Autodesk Inventor part; units mm, degrees
ref_plane "Work Plane1" through (-29.1, -14.5, 2.4) normal (0, 0, -1) x (0, 1, 0)
ref_plane "Work Plane2" through (-13.8999, -10.5497, 2.25) normal (0, 0, -1) x (0, 1, 0)
ref_plane "YZ Plane" through (0, 0, 0) normal (1, 0, 0) x (0, 1, 0)
ref_plane "Work Plane1" through (-29.1, -14.5, 2.4) normal (0, 0, -1) x (0, 1, 0)
ref_plane "Work Plane2" through (-13.8999, -10.5497, 2.25) normal (0, 0, -1) x (0, 1, 0)
sketch "Sketch1" plane through (0, 0, 0) normal (0, 0, 1) x (1, 0, 0)
  line L0 (-34.86, 0) -> (34.86, 0) construction
  line L1 (0, -34.86) -> (0, 34.86) construction
  line L2 (0, 0) -> (11.1575, 11.1575) construction
  line L3 (0, 0) -> (15.7791, 0) construction
  line L4 (0, 24.9) -> (16.8009, 24.9)
  line L5 (16.8009, 24.9) -> (16.8009, 21.2415)
  line L6 (16.8009, 21.2415) -> (19.0212, 19.0212)
  line L7 (24.9, 0) -> (24.9, 16.8009)
  line L8 (24.9, 16.8009) -> (21.2415, 16.8009)
  line L9 (21.2415, 16.8009) -> (19.0212, 19.0212)
  line L10 (0, -24.9) -> (16.8009, -24.9)
  line L11 (16.8009, -24.9) -> (16.8009, -21.2415)
  line L12 (16.8009, -21.2415) -> (19.0212, -19.0212)
  line L13 (24.9, 0) -> (24.9, -16.8009)
  line L14 (24.9, -16.8009) -> (21.2415, -16.8009)
  line L15 (21.2415, -16.8009) -> (19.0212, -19.0212)
  line L16 (0, 24.9) -> (-16.8009, 24.9)
  line L17 (-16.8009, 24.9) -> (-16.8009, 21.2415)
  line L18 (-16.8009, 21.2415) -> (-19.0212, 19.0212)
  line L19 (-24.9, 16.8009) -> (-21.2415, 16.8009)
  line L20 (-21.2415, 16.8009) -> (-19.0212, 19.0212)
  line L21 (0, -24.9) -> (-16.8009, -24.9)
  line L22 (-16.8009, -24.9) -> (-16.8009, -21.2415)
  line L23 (-16.8009, -21.2415) -> (-19.0212, -19.0212)
  line L24 (-21.2415, -16.8009) -> (-19.0212, -19.0212)
  line L25 (-24.9, -16.8009) -> (-21.2415, -16.8009)
  line L26 (-24.9, 0) -> (-24.9, -16.8009)
  line L27 (-24.9, 0) -> (-24.9, 16.8009)
  circle A0 centre (0, 0) radius 5
  dimension "d0" = 45
  dimension "d2" = 24.9
  dimension "d3" = 3.14
  dimension "d4" = 26.9
  dimension "d5" = 10
extrude "Extrusion1" add sketch "Sketch1" along normal up to surface (2.25 mm away)
sketch "Sketch5" plane through (0, 0, 0) normal (0, 0, -1) x (-1, 0, 0)
  circle A0 centre (-9.7, 10) radius 1.4
  circle A1 centre (-9.7, -10) radius 1.4
  circle A2 centre (13.8, 0) radius 1.4
  circle A3 centre (-10, 6.9) radius 0.75
  circle A4 centre (10, 6.9) radius 1.25
  point P0 (0, 0)
hole "Hole1" at (9.7, -10, 0) at (9.7, 10, 0) direction (0, 0, 1) diameter 3.3 depth 12 tip angle 118
sketch "Sketch6" plane through (-16.8009, 24.9, 2.25) normal (0, 0, 1) x (1, 0, 0)
  circle A0 centre (26.5009, -34.9) radius 1.65 construction
  circle A1 centre (26.5009, -14.9) radius 1.65 construction
  circle A2 centre (16.8009, -24.9) radius 5 construction
  line L0 (33.6017, -3.6585) -> (33.6017, 0) construction
  line L1 (33.6017, 0) -> (0, 0) construction
  line L2 (0, 0) -> (0, -3.6585) construction
  line L3 (0, -3.6585) -> (-4.4406, -8.0991) construction
  line L4 (-4.4406, -8.0991) -> (-8.0991, -8.0991) construction
  line L5 (-8.0991, -8.0991) -> (-8.0991, -41.7009) construction
  line L6 (-8.0991, -41.7009) -> (-4.4406, -41.7009) construction
  line L7 (-4.4406, -41.7009) -> (0, -46.1415) construction
  line L8 (0, -46.1415) -> (0, -49.8) construction
  line L9 (0, -49.8) -> (33.6017, -49.8) construction
  line L10 (33.6017, -49.8) -> (33.6017, -46.1415) construction
  line L11 (33.6017, -46.1415) -> (38.0423, -41.7009) construction
  line L12 (38.0423, -41.7009) -> (41.7009, -41.7009) construction
  line L13 (41.7009, -41.7009) -> (41.7009, -8.0991) construction
  line L14 (41.7009, -8.0991) -> (38.0423, -8.0991) construction
  line L15 (38.0423, -8.0991) -> (33.6017, -3.6585) construction
  line L16 (33.7009, -14.9) -> (-0.0991, -14.9)
  line L17 (33.7009, -16.55) -> (-0.0991, -16.55)
  line L18 (-0.0991, -13.25) -> (33.7009, -13.25)
  arc A3 (33.7009, -16.55) -> (33.7009, -13.25) centre (33.7009, -14.9) ccw
  arc A4 (-0.0991, -13.25) -> (-0.0991, -16.55) centre (-0.0991, -14.9) ccw
  line L19 (-8.0991, -41.7009) -> (-8.0991, -8.0991) construction
  line L20 (-8.0991, -24.9) -> (41.7009, -24.9) construction
  line L21 (41.7009, -8.0991) -> (41.7009, -41.7009) construction
  circle A5 centre (26.5009, -34.9) radius 1.65 construction
  line L22 (33.7009, -34.9) -> (-0.0991, -34.9)
  line L23 (33.7009, -33.25) -> (-0.0991, -33.25)
  line L24 (-0.0991, -36.55) -> (33.7009, -36.55)
  arc A6 (33.7009, -36.55) -> (33.7009, -33.25) centre (33.7009, -34.9) ccw
  arc A7 (-0.0991, -33.25) -> (-0.0991, -36.55) centre (-0.0991, -34.9) ccw
  point P0 (16.8009, -24.9)
  point P1 (16.8009, -14.9)
  point P2 (16.8009, -34.9)
  dimension "d25" = 8
  dimension "d26" = 8
extrude "Extrusion5" cut sketch "Sketch6" against normal through all
sketch "Skizze7" plane through (-16.8009, 24.9, 2.25) normal (0, 0, 1) x (1, 0, 0)
  line L0 (33.7009, -16.55) -> (-0.0991, -16.55) construction
  arc A0 (-0.0991, -13.25) -> (-0.0991, -16.55) centre (-0.0991, -14.9) ccw construction
  line L1 (-0.0991, -13.25) -> (33.7009, -13.25) construction
  arc A1 (33.7009, -16.55) -> (33.7009, -13.25) centre (33.7009, -14.9) ccw construction
  line L2 (-0.0991, -33.25) -> (33.7009, -33.25) construction
  arc A2 (33.7009, -36.55) -> (33.7009, -33.25) centre (33.7009, -34.9) ccw construction
  line L3 (33.7009, -36.55) -> (-0.0991, -36.55) construction
  arc A3 (-0.0991, -33.25) -> (-0.0991, -36.55) centre (-0.0991, -34.9) ccw construction
  circle A4 centre (16.8009, -24.9) radius 5 construction
  line L4 (33.6017, -3.6585) -> (33.6017, 0)
  line L5 (33.6017, 0) -> (0, 0) construction
  line L6 (0, 0) -> (0, -3.6585)
  line L7 (0, -3.6585) -> (-4.4406, -8.0991)
  line L8 (-4.4406, -8.0991) -> (-8.0991, -8.0991)
  line L9 (-8.0991, -8.0991) -> (-8.0991, -41.7009) construction
  line L10 (-8.0991, -41.7009) -> (-4.4406, -41.7009)
  line L11 (-4.4406, -41.7009) -> (0, -46.1415)
  line L12 (0, -46.1415) -> (0, -49.8)
  line L13 (0, -49.8) -> (33.6017, -49.8) construction
  line L14 (33.6017, -49.8) -> (33.6017, -46.1415)
  line L15 (33.6017, -46.1415) -> (38.0423, -41.7009)
  line L16 (38.0423, -41.7009) -> (41.7009, -41.7009)
  line L17 (41.7009, -41.7009) -> (41.7009, -8.0991) construction
  line L18 (41.7009, -8.0991) -> (38.0423, -8.0991)
  line L19 (38.0423, -8.0991) -> (33.6017, -3.6585)
  line L20 (-0.2, 0.2) -> (33.8017, 0.2) construction
  line L21 (33.8017, 0.2) -> (33.8017, -3.5757)
  line L22 (33.8017, -3.5757) -> (38.1252, -7.8991)
  line L23 (38.1252, -7.8991) -> (41.9009, -7.8991)
  line L24 (41.9009, -7.8991) -> (41.9009, -41.9009) construction
  line L25 (41.9009, -41.9009) -> (38.1252, -41.9009)
  line L26 (38.1252, -41.9009) -> (33.8017, -46.2243)
  line L27 (33.8017, -46.2243) -> (33.8017, -50)
  line L28 (33.8017, -50) -> (-0.2, -50) construction
  line L29 (-0.2, -50) -> (-0.2, -46.2243)
  line L30 (-0.2, -46.2243) -> (-4.5235, -41.9009)
  line L31 (-4.5235, -41.9009) -> (-8.2991, -41.9009)
  line L32 (-8.2991, -41.9009) -> (-8.2991, -7.8991) construction
  line L33 (-8.2991, -7.8991) -> (-4.5235, -7.8991)
  line L34 (-4.5235, -7.8991) -> (-0.2, -3.5757)
  line L35 (-0.2, -3.5757) -> (-0.2, 0.2)
  line L36 (33.6017, 0) -> (0, 0)
  line L37 (0, 0) -> (-0.2, 0)
  line L38 (-8.0991, -41.7009) -> (-8.0991, -8.0991)
  line L39 (-8.0991, -8.0991) -> (-8.0991, -7.8991)
  line L40 (33.6017, 0) -> (33.6017, -3.6585)
  line L41 (33.6017, 0) -> (33.8017, 0)
  line L42 (41.7009, -8.0991) -> (41.7009, -7.8991)
  line L43 (41.7009, -41.7009) -> (38.0423, -41.7009)
  line L44 (41.7009, -41.7009) -> (41.7009, -41.9009)
  line L45 (33.6017, -49.8) -> (33.8017, -49.8)
  line L46 (0, -49.8) -> (0, -46.1415)
  line L47 (0, -49.8) -> (-0.2, -49.8)
  line L48 (-8.0991, -41.7009) -> (-8.0991, -41.9009)
  point P0 (16.8009, -24.9)
  dimension "d29" = 0.2
extrude "IM_offset" add sketch "Skizze7" against normal up to surface (2.25 mm away)
properties part number "20_Cube_insert_Sample_holder"
Here's how the part is built. I have some questions about the finished solid (model axes, mm). A direction names the side the tool comes from. Round coordinates to 2 decimals unless told otherwise and drop trailing zeros. Write each loop counter-clockwise with the first axis right and the second up, starting at its lowest first coordinate (ties: lowest second). Pieces come first, ordered by that corner, then holes. Notation, with made-up numbers: (-7.75, 11.5) -> (23.25, 11.5) arc R19 ccw to (23.25, 45.5) -> close; hole circle Ø1 at (-18.75, -34.75). An arc over 180 degrees is marked (long way). One line per item, written item: value.
1) Suppose I cut it at D-D on x = -12. List the corners of the cut face in (y, z) for me, plus the area to 3 significant figures.
Filled sheet:
outline: (-24.9, 0) -> (-11.65, 0) -> (-11.65, 2.25) -> (-24.9, 2.25) -> close; (-8.35, 0) -> (8.35, 0) -> (8.35, 2.25) -> (-8.35, 2.25) -> close; (11.65, 0) -> (24.9, 0) -> (24.9, 2.25) -> (11.65, 2.25) -> close
area: 97.2 mm2
2) We'd pull the mould along Y, two halves only. Please class faces 6 (the face through (23, -17.001, 1)), 7 (the face through (-17.001, 23, 1)), 8 (the face through (0, 8.35, 1)): released by +Y, released by -Y, zero draft, split by the parting line, or undercut.
Filled sheet:
face 6: released by -Y
face 7: zero draft
face 8: undercut
3) For faces 1 (the face through (18.55, -10.04, 1.14)), 2 (the face through (0, 6, 2.25)), 3 (the face through (-17.001, -23, 1)), 4 (the face through (17.001, 23, 1)), 5 (the face through (17.001, -23, 1)), which set-ups out of +Z, -Z, +X, -X, +Y, -Y let a thin tool reach every point of the face, with its end or its side?
Filled sheet:
face 1: +Z, -Z
face 2: +Z, +X, -X, +Y, -Y
face 3: +Z, -Z, -X, -Y
face 4: +Z, -Z, +X, +Y
face 5: +Z, -Z, +X, -Y
4) Suppose I cut it at A-A on x = 0. List the corners of the cut face in (y, z) for me, plus the area to 3 significant figures.
Filled sheet:
outline: (-24.9, 0) -> (-11.65, 0) -> (-11.65, 2.25) -> (-24.9, 2.25) -> close; (-8.35, 0) -> (-5, 0) -> (-5, 2.25) -> (-8.35, 2.25) -> close; (5, 0) -> (8.35, 0) -> (8.35, 2.25) -> (5, 2.25) -> close; (11.65, 0) -> (24.9, 0) -> (24.9, 2.25) -> (11.65, 2.25) -> close
area: 74.7 mm2
5) Suppose I cut it at C-C on z = 1.3. List the corners of the cut face in (x, y) for me.
Filled sheet:
outline: (-24.9, -17) -> (-21.32, -17) -> (-17, -21.32) -> (-17, -24.9) -> (17, -24.9) -> (17, -21.32) -> (21.32, -17) -> (24.9, -17) -> (24.9, 17) -> (21.32, 17) -> (17, 21.32) -> (17, 24.9) -> (-17, 24.9) -> (-17, 21.32) -> (-21.32, 17) -> (-24.9, 17) -> close; hole (-16.9, -11.65) -> (16.9, -11.65) arc R1.65 ccw to (16.9, -8.35) -> (-16.9, -8.35) arc R1.65 ccw to start; hole (-16.9, 8.35) -> (16.9, 8.35) arc R1.65 ccw to (16.9, 11.65) -> (-16.9, 11.65) arc R1.65 ccw to start; hole circle Ø10 at (0, 0)
6) If I drill on line 1 (Y direction, x = 0, z = 1.25); line 2 (Y direction, x = -16.5, z = 1.95); line 3 (Y direction, x = -3, z = 2.2), over which ranges is the centre line in solid material (lowest first)? Write a range as [from, to].
Filled sheet:
line 1: y = [-24.9, -11.65], [-8.35, -5], [5, 8.35], [11.65, 24.9]
line 2: y = [-24.9, -11.65], [-8.35, 8.35], [11.65, 24.9]
line 3: y = [-24.9, -11.65], [-8.35, -4], [4, 8.35], [11.65, 24.9]
7) I'm going to push flat-ended pins straight in: pin 1 Ø1 at (y, z) = (18.5, 1.5) entering from +X; pin 2 Ø0.7 at (y, z) = (23, 1) entering from +X; pin 3 Ø1.1 at (x, z) = (22.5, 1.5) entering from +Y. Where does each tip first touch, or does it pass through?
Filled sheet:
pin 1: stops at x = 20.33
pin 2: stops at x = 17
pin 3: stops at y = 17
8) Suppose I cut it at B-B on y = 0. List the corners of the cut face in (x, z) for me, plus the area to 4 significant figures.
Filled sheet:
outline: (-24.9, 0) -> (-5, 0) -> (-5, 2.25) -> (-24.9, 2.25) -> close; (5, 0) -> (24.9, 0) -> (24.9, 2.25) -> (5, 2.25) -> close
area: 89.55 mm2
